Read the model definition and answer for the solid it produces. Units are mm, in the model's axes. Face numbers are marked on the shaded views. A direction names the side the tool comes from. Give positions to 0.01 mm unless a question says otherwise; leave off trailing zeros. Order: outer loops, then holes, each group sorted by start corner. A loop starts at its lowest first (then second) coordinate and runs counter-clockwise, first axis right, second up.
Item 1: A cutting plane is placed at B-B (z = -6.5). Write down the section's boundary in (x, y) (3 decimals).
Item 2: Given pin 1 Ø4.5 at (x, y) = (-28, -2) entering from -Z; pin 2 Ø4 at (y, z) = (-2.5, -30) entering from +X; pin 3 Ø9.5 at (y, z) = (3.5, -28.5) entering from -X, each flat-ended and moving along its own axis, determine where each tip first touches the part or whether it passes through.
Item 3: Which of the six approach directions +Z, -Z, +X, -X, +Y, -Y give full straight-line access (tool end or side, diameter ignored) to the marked faces 1, 2, 3, 4 and 5?
Item 4: A cutting plane is placed at A-A (x = 0). Write down the section's boundary in (y, z).
Item 5: The mould has two halves that part along X. Classify the marked faces 6, 7 and 8: +X half, -X half, draft (parallel to the pull), parting line (faces both ways), or undercut.
Item 6: A cutting plane is placed at C-C (y = -13). Write down the section's boundary in (x, z) (3 decimals), plus the area to 3 significant figures.
Item 7: Find the intervals of material crossed by line 1 along X through (y, z) = (3, -17.5) (3 decimals); line 2 along X through (y, z) = (-3, -25); line 3 along X through (y, z) = (-1, -13.5) (3 decimals), in increasing order.
Item 8: A cutting plane is placed at D-D (z = -30). Write down the section's boundary in (x, y), plus the area to 3 significant figures.
from build123d import *

# Parameters (mm, degrees)
F0_W      = 68.95
F0_H      = 31.6738
F1_DEPTH  = 21
F2_W      = 39.7002
F2_H      = 31.6738
F3_DEPTH  = 11
F4_R      = 6.4262
F4_R_2    = 2.794
F5_DEPTH  = 2
F6_R      = 3
F7_DEPTH  = 34.001
F9_DEPTH  = 10
F11_DEPTH = 31.6748
F12_W     = 39.7002
F12_H     = 2
F13_DEPTH = 3
F14_R     = 2.5
F15_DEPTH = 34.001
F17_DEPTH = 25.001
F18_R     = 2
F19_R     = 2


with BuildPart() as f1:
    # F0 (on Top) → F1 (new body)
    with BuildSketch(Plane.XY):
        Rectangle(F0_W, F0_H)
    extrude(amount=-F1_DEPTH)

    # F2 (on face) → F3 (join)
    with BuildSketch(Plane(origin=(0, 0, -21), x_dir=(1, 0, 0), z_dir=(0, 0, -1))):
        Rectangle(F2_W, F2_H)
    extrude(amount=F3_DEPTH)

    # F4 (on face) → F5 (join)
    with BuildSketch(Plane.XY):
        with Locations((-26.475, 0)):
            Circle(F4_R)
        with Locations((-26.475, 0)):
            Circle(F4_R_2, mode=Mode.SUBTRACT)
        with Locations((26.475, 0)):
            Circle(F4_R)
    extrude(amount=F5_DEPTH)

    # F6 (on face) → F7 (cut, through all)
    with BuildSketch(Plane.XY.offset(2)):
        with Locations((-26.475, 0)):
            Circle(F6_R)
        with Locations((26.475, 0)):
            Circle(F6_R)
    extrude(amount=-F7_DEPTH, mode=Mode.SUBTRACT)

    # F8 (on face) → F9 (cut)
    with BuildSketch(Plane(origin=(0, 0, -21), x_dir=(1, 0, 0), z_dir=(0, 0, -1))):
        Polygon((-26.475, 5.196152), (-30.975, 2.598076), (-30.975, -2.598076), (-26.475, -5.196152), (-21.975, -2.598076), (-21.975, 2.598076), align=None)
        Polygon((26.475, -5.196152), (30.975, -2.598076), (30.975, 2.598076), (26.475, 5.196152), (21.975, 2.598076), (21.975, -2.598076), align=None)
    extrude(amount=-F9_DEPTH, mode=Mode.SUBTRACT)

    # F10 (on face) → F11 (cut, through all)
    with BuildSketch(Plane.XZ.offset(15.8369)):
        with BuildLine():
            Line((4.5, -23), (4.5, -16.393596))
            ThreePointArc((4.5, -16.393596), (13.518506, -10.307764), (17, 0))
            Line((17, 0), (-17, 0))
            ThreePointArc((-17, 0), (-13.518506, -10.307764), (-4.5, -16.393596))
            Line((-4.5, -16.393596), (-4.5, -23))
            Line((-4.5, -23), (4.5, -23))
        make_face()
    extrude(amount=-F11_DEPTH, mode=Mode.SUBTRACT)

    # F12 (on face) → F13 (join)
    with BuildSketch(Plane(origin=(0, 0, -32), x_dir=(1, 0, 0), z_dir=(0, 0, -1))):
        with Locations((0, 14.8369)):
            Rectangle(F12_W, F12_H)
        with Locations((0, -14.8369)):
            Rectangle(F12_W, F12_H)
    extrude(amount=F13_DEPTH)

    # F14 (on face) → F15 (cut, through all)
    with BuildSketch(Plane(origin=(0, 0, -32), x_dir=(1, 0, 0), z_dir=(0, 0, -1))):
        with Locations((-6.5, 3.752777)):
            Circle(F14_R)
        with Locations((6.5, 3.752777)):
            Circle(F14_R)
        with Locations((0, -7.505553)):
            Circle(F14_R)
    extrude(amount=-F15_DEPTH, mode=Mode.SUBTRACT)

    # F16 (on face) → F17 (cut, through all)
    with BuildSketch(Plane.XY.offset(-23)):
        with BuildLine():
            ThreePointArc((-6.5, 1.747223), (-12, -3.752777), (-6.5, -9.252777))
            Line((-6.5, -9.252777), (6.5, -9.252777))
            ThreePointArc((6.5, -9.252777), (12, -3.752777), (6.5, 1.747223))
            Line((6.5, 1.747223), (-6.5, 1.747223))
        make_face()
    extrude(amount=F17_DEPTH, mode=Mode.SUBTRACT)

    # F18
    f18_edges = [f1.edges().sort_by_distance(p)[0] for p in [
        (-34.475, -15.8369, -10.5),
        (34.475, -15.8369, -10.5),
        (34.475, 15.8369, -10.5),
        (-34.475, 15.8369, -10.5),
    ]]
    fillet(f18_edges, radius=F18_R)

    # F19
    f19_edges = [f1.edges().sort_by_distance(p)[0] for p in [
        (-19.8501, 0, -21),
        (19.8501, 0, -21),
    ]]
    fillet(f19_edges, radius=F19_R)


solid = f1.part
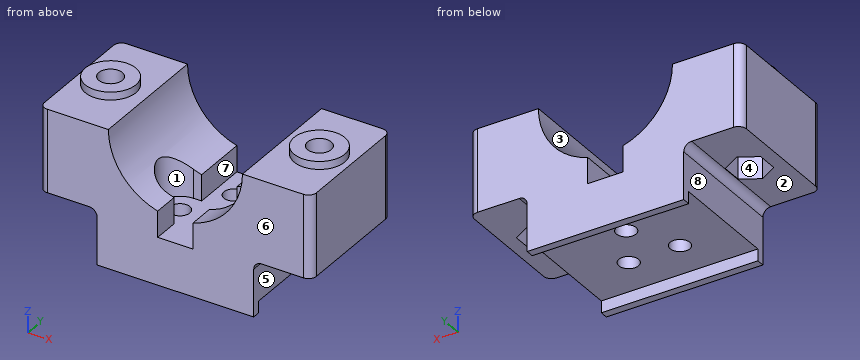
Response values:
1. outline: (-34.475, -13.837) arc R2 ccw to (-32.475, -15.837) - (-15.708, -15.837) - (-15.708, 15.837) - (-32.475, 15.837) arc R2 ccw to (-34.475, 13.837) - close; (15.708, -15.837) - (32.475, -15.837) arc R2 ccw to (34.475, -13.837) - (34.475, 13.837) arc R2 ccw to (32.475, 15.837) - (15.708, 15.837) - close; hole circle Ø6 at (-26.475, 0); hole circle Ø6 at (26.475, 0)
2. pin 1: stops at z = -21
2. pin 2: stops at x = 19.85
2. pin 3: stops at x = -19.85
3. face 1: +Z
3. face 2: -Z, -X, +Y, -Y
3. face 3: +Z, +Y, -Y
3. face 4: -Z
3. face 5: -Z, +X, +Y, -Y
4. outline: (-15.84, -35) - (-13.84, -35) - (-13.84, -32) - (5.01, -32) - (5.01, -23) - (-15.84, -23) - close; (10.01, -32) - (13.84, -32) - (13.84, -35) - (15.84, -35) - (15.84, -23) - (10.01, -23) - close
5. face 6: draft
5. face 7: undercut
5. face 8: -X half
6. outline: (-34.475, -21) - (-21.85, -21) arc R2 cw to (-19.85, -23) - (-19.85, -32) - (19.85, -32) - (19.85, -23) arc R2 cw to (21.85, -21) - (34.475, -21) - (34.475, 0) - (17, 0) arc R17 cw to (4.5, -16.394) - (4.5, -23) - (-4.5, -23) - (-4.5, -16.394) arc R17 cw to (-17, 0) - (-34.475, 0) - close
6. area: 1,380 mm2
7. line 1: x = -34.475 to -30.279, -22.671 to -4.5, 4.5 to 22.671, 30.279 to 34.475
7. line 2: x = -19.85 to -8.88, -4.12 to 4.12, 8.88 to 19.85
7. line 3: x = -34.475 to -30.975, -21.975 to -11.262, 11.262 to 21.975, 30.975 to 34.475
8. outline: (-19.85, -15.84) - (19.85, -15.84) - (19.85, 15.84) - (-19.85, 15.84) - close; hole circle Ø5 at (-6.5, -3.75); hole circle Ø5 at (0, 7.51); hole circle Ø5 at (6.5, -3.75)
8. area: 1,200 mm2
